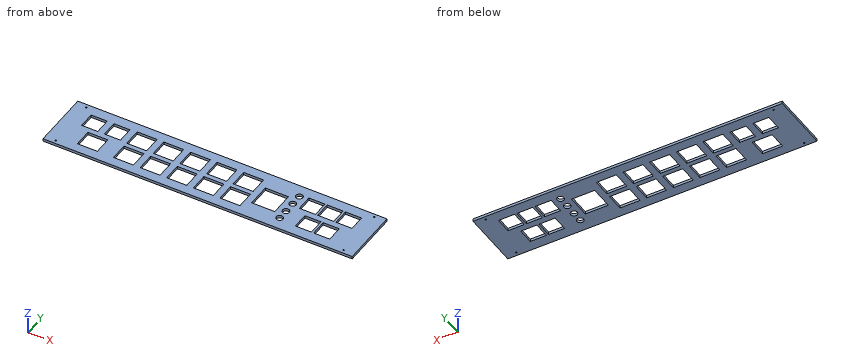
from build123d import *

# Parameters (mm, degrees)
F0_W     = 693
F0_H     = 131.4
F0_R     = 1.575
F0_W_2   = 44.7
F0_H_2   = 39.7
F0_R_2   = 7.5
F0_W_3   = 36
F0_H_3   = 36
F0_W_4   = 51.7
F0_H_4   = 51.7
F1_DEPTH = 6


with BuildPart() as f1:
    # F0 (on Top) → F1 (new body)
    with BuildSketch(Plane.XY):
        with Locations((-257.70224, 23.026403)):
            Rectangle(F0_W, F0_H)
        with Locations((-580.20224, -34.673597)):
            Circle(F0_R, mode=Mode.SUBTRACT)
        with Locations((-517.20224, -1.823597)):
            Rectangle(F0_W_2, F0_H_2, mode=Mode.SUBTRACT)
        with Locations((-436.35224, -1.823597)):
            Rectangle(F0_W_2, F0_H_2, mode=Mode.SUBTRACT)
        with Locations((-376.65224, -1.823597)):
            Rectangle(F0_W_2, F0_H_2, mode=Mode.SUBTRACT)
        with Locations((-316.95224, -1.823597)):
            Rectangle(F0_W_2, F0_H_2, mode=Mode.SUBTRACT)
        with Locations((-90.60224, -14.248597)):
            Circle(F0_R_2, mode=Mode.SUBTRACT)
        with Locations((64.79776, -34.673597)):
            Circle(F0_R, mode=Mode.SUBTRACT)
        with Locations((-257.25224, -1.823597)):
            Rectangle(F0_W_2, F0_H_2, mode=Mode.SUBTRACT)
        with Locations((-197.55224, -1.823597)):
            Rectangle(F0_W_2, F0_H_2, mode=Mode.SUBTRACT)
        with Locations((-90.60224, 9.505447)):
            Circle(F0_R_2, mode=Mode.SUBTRACT)
        with Locations((-34.20224, -1.823597)):
            Rectangle(F0_W_3, F0_H_3, mode=Mode.SUBTRACT)
        with Locations((6.79776, -1.823597)):
            Rectangle(F0_W_3, F0_H_3, mode=Mode.SUBTRACT)
        with Locations((-542.70224, 47.876403)):
            Rectangle(F0_W_3, F0_H_3, mode=Mode.SUBTRACT)
        with Locations((-491.70224, 47.876403)):
            Rectangle(F0_W_3, F0_H_3, mode=Mode.SUBTRACT)
        with Locations((-436.35224, 47.876403)):
            Rectangle(F0_W_2, F0_H_2, mode=Mode.SUBTRACT)
        with Locations((-376.65224, 47.876403)):
            Rectangle(F0_W_2, F0_H_2, mode=Mode.SUBTRACT)
        with Locations((-316.95224, 47.876403)):
            Rectangle(F0_W_2, F0_H_2, mode=Mode.SUBTRACT)
        with Locations((-580.20224, 80.726403)):
            Circle(F0_R, mode=Mode.SUBTRACT)
        with Locations((-134.35224, 23.026403)):
            Rectangle(F0_W_4, F0_H_4, mode=Mode.SUBTRACT)
        with Locations((-90.60224, 35.136569)):
            Circle(F0_R_2, mode=Mode.SUBTRACT)
        with Locations((-257.25224, 47.876403)):
            Rectangle(F0_W_2, F0_H_2, mode=Mode.SUBTRACT)
        with Locations((-197.55224, 47.876403)):
            Rectangle(F0_W_2, F0_H_2, mode=Mode.SUBTRACT)
        with Locations((-54.70224, 47.876403)):
            Rectangle(F0_W_3, F0_H_3, mode=Mode.SUBTRACT)
        with Locations((-13.70224, 47.876403)):
            Rectangle(F0_W_3, F0_H_3, mode=Mode.SUBTRACT)
        with Locations((27.29776, 47.876403)):
            Rectangle(F0_W_3, F0_H_3, mode=Mode.SUBTRACT)
        with Locations((-90.60224, 60.301403)):
            Circle(F0_R_2, mode=Mode.SUBTRACT)
        with Locations((64.79776, 80.726403)):
            Circle(F0_R, mode=Mode.SUBTRACT)
    extrude(amount=F1_DEPTH)


solid = f1.part
Design review of the part built by this model. Coordinates are the model's own, in mm. Round coordinates to 2 decimals unless told otherwise and drop trailing zeros. Loops run counter-clockwise (first coordinate to the right, second up) from the corner with the lowest first, then second, coordinate; pieces in that order, holes last. Notation, with made-up numbers: (-23, -17.5) - (-16, -17.5) arc R18 ccw to (-16, -1.5) - close; hole circle Ø1 at (63, 24.25). An arc over 180 degrees is marked (long way). One line per question, with ' | ' between items.
1. For L1, parallel to Y at x = -241, z = 1.3; L2, parallel to Y at x = -532, z = 4.95; L3, parallel to Y at x = 26.5, z = 0.9, list the stretches that pass through material, from the lowest coordinate up. Write a range as [from, to].
Results are:
L1: y = [-42.67, -21.67], [18.03, 28.03], [67.73, 88.73] | L2: y = [-42.67, -21.67], [18.03, 29.88], [65.88, 88.73] | L3: y = [-42.67, 29.88], [65.88, 88.73]
2. We need section B-B, the plane z = 1.95. State how many separate pieces and enclosed holes the cut face has, and give its area (3 significant figures).
Results are:
separate pieces: 1 | enclosed holes: 27 | area: 59,100 mm²
3. We need section A-A, the plane x = -433.5. State the section outline as (y, z) points.
Results are:
outline: (-42.67, 0) - (-21.67, 0) - (-21.67, 6) - (-42.67, 6) - close; (18.03, 0) - (28.03, 0) - (28.03, 6) - (18.03, 6) - close; (67.73, 0) - (88.73, 0) - (88.73, 6) - (67.73, 6) - close
